Source: CAD feature listing. Evaluate the final solid. Frame: model axes, mm. Round coordinates to 2 decimals unless told otherwise and drop trailing zeros. Write each loop counter-clockwise with the first axis right and the second up, starting at its lowest first coordinate (ties: lowest second). Pieces come first, ordered by that corner, then holes.
```python
from build123d import *

# Parameters (mm, degrees)
STOCK_BOXV2_1_START     = -19.05
STOCK_BOXV2_1_OUTLINE_W = 19.05
STOCK_BOXV2_1_OUTLINE_H = 488.95
STOCK_BOXV2_1_DEPTH     = 609.6
SKETCH1_R               = 25.4
CUT_EXTRUDE1_DEPTH      = 19.05


# Read off the part's stored shape, not the designer's step: Stock-boxV2-1
with BuildPart() as part:
    # Stock-boxV2-1 outline → Stock-boxV2-1 (new body)
    with BuildSketch(Plane(origin=(0, 0, 0), x_dir=(1, 0, 0), z_dir=(0, 1, 0)).offset(STOCK_BOXV2_1_START)):
        with Locations((-517.525, 0)):
            Rectangle(STOCK_BOXV2_1_OUTLINE_W, STOCK_BOXV2_1_OUTLINE_H)
    extrude(amount=STOCK_BOXV2_1_DEPTH)

    # Sketch1 → Cut-Extrude1 (cut)
    with BuildSketch(Plane(origin=(-508, 0, 0), x_dir=(0, 0, -1), z_dir=(1, 0, 0))):
        with Locations((168.275, 514.35)):
            Circle(SKETCH1_R)
    extrude(amount=-CUT_EXTRUDE1_DEPTH, mode=Mode.SUBTRACT)


solid = part.part
```
Q1. Mould query, pull axis Y, two halves, no side actions, for faces 1 (the face through (-517.392, 531.517, -149.554)), 2 (the face through (-518, 590.55, -3)), 3 (the face through (-518, 281, 244.475)). Classes: pulls with the +Y half, pulls with the -Y half, needs draft (parallel to the pull), parting line crosses it, or undercut.
Q2. Section query A-A, the plane y = 514.35. Output: boundary loops of the cut face in (x, z) (3 decimals), and give its area (3 significant figures).
Q3. Line query: line 1 (Z direction, x = -518, y = 506) (3 decimals); line 2 (Z direction, x = -523, y = 500) (3 decimals). Output: solid intervals per line, ascending.
Filled in:
1. face 1: undercut
1. face 2: pulls with the +Y half
1. face 3: needs draft
2. outline: (-527.05, -244.475) - (-508, -244.475) - (-508, -193.675) - (-527.05, -193.675) - close; (-527.05, -142.875) - (-508, -142.875) - (-508, 244.475) - (-527.05, 244.475) - close
2. area: 8,350 mm2
3. line 1: z = -244.475 to -192.263, -144.287 to 244.475
3. line 2: z = -244.475 to -189.233, -147.317 to 244.475
